The listing builds one solid part. Answer for the finished solid, in the listing's coordinates (mm). Face numbers are marked on the shaded views. A direction names the side the tool comes from. Give positions to 0.01 mm unless a question says otherwise; leave off trailing zeros. Write each loop counter-clockwise with the first axis right and the second up, starting at its lowest first coordinate (ties: lowest second). Pieces come first, ordered by that corner, then holes.
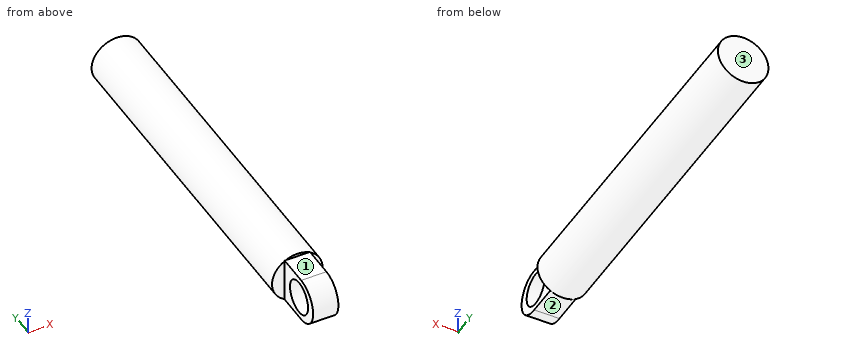
```python
from build123d import *

# Parameters (mm, degrees)
SKETCH5_R           = 14.989713258
BOSS_EXTRUDE3_DEPTH = 200
BOSS_EXTRUDE4_DEPTH = 7.5
SKETCH7_R           = 9.985206203
CUT_EXTRUDE2_DEPTH  = 20


with BuildPart() as part:
    # Sketch5 → Boss-Extrude3 (new body)
    with BuildSketch(Plane(origin=(0, 0, 0), x_dir=(1, 0, 0), z_dir=(0, 1, 0))):
        Circle(SKETCH5_R)
    extrude(amount=BOSS_EXTRUDE3_DEPTH)

    # Sketch6 → Boss-Extrude4 (add, symmetric)
    with BuildSketch(Plane(origin=(0, 0, 0), x_dir=(0, -1, 0), z_dir=(-1, 0, 0))):
        with BuildLine():
            Line((0, 13.292901933), (18.33265387, 13.292901933))
            ThreePointArc((18.33265387, 13.292901933), (31.584492176, -0.298051084), (17.663099627, -13.202315957))
            Line((17.663099627, -13.202315957), (0, -13.202315957))
            Line((0, -13.202315957), (0, 13.292901933))
        make_face()
    extrude(amount=BOSS_EXTRUDE4_DEPTH, both=True)

    # Sketch7 → Cut-Extrude2 (cut, symmetric)
    with BuildSketch(Plane(origin=(7.5, 0, 0), x_dir=(0, 0, -1), z_dir=(1, 0, 0))):
        with Locations((0, -15.988279057)):
            Circle(SKETCH7_R)
    extrude(amount=CUT_EXTRUDE2_DEPTH, both=True, mode=Mode.SUBTRACT)


solid = part.part
```
Item 1: Each of these flat-tipped pins is pushed along its axis until it touches: P1, Ø1, axis at x = -7, z = 8.5, coming from the -Y side; P2, Ø12, axis at y = 37.5, z = 10, coming from the -X side; P3, Ø6, axis at x = -12.5, z = 0.5, coming from the -Y side. Where does it stop, or does it pass through?
Conclusion:
P1: stops at y = -28.93
P2: stops at x = -14.45
P3: stops at y = 0
Item 2: A cutting plane is placed at D-D, the plane x = -11.5. Give the vertices of the cut face in (y, z), plus the area to 3 significant figures.
Conclusion:
outline: (0, -9.61) - (200, -9.61) - (200, 9.61) - (0, 9.61) - close
area: 3,850 mm2
Item 3: Consider probe 1 along Y at (x, z) = (-2.5, 0); probe 2 along Z at (x, y) = (13, 137); probe 3 along Y at (x, z) = (-4, -5). Determine where each line is inside the solid, lowest interval first.
Conclusion:
probe 1: y = -31.59 to -25.97, -6 to 200
probe 2: z = -7.46 to 7.46
probe 3: y = -30.59 to -24.63, -7.35 to 200
Item 4: A cutting plane is placed at A-A, the plane x = 1.75. Give the vertices of the cut face in (y, z).
Conclusion:
outline: (-18.33, 13.29) arc R13.26 ccw (long way) to (-17.66, -13.2) - (0, -13.2) - (0, -14.89) - (200, -14.89) - (200, 14.89) - (0, 14.89) - (0, 13.29) - close; hole circle Ø19.97 at (-15.99, 0)
Item 5: A cutting plane is placed at C-C, the plane y = 106.5. Give the vertices of the cut face in (x, z), plus the area to 3 significant figures.
Conclusion:
outline: circle Ø29.98 at (0, 0)
area: 706 mm2
Item 6: Which of the six approach directions +Z, -Z, +X, -X, +Y, -Y give full straight-line access (tool end or side, diameter ignored) to the marked faces 1, 2 and 3?
Conclusion:
face 1: +Z, +X, -X, -Y
face 2: -Z, +X, -X, -Y
face 3: +Z, -Z, +X, -X, +Y
Item 7: A cutting plane is placed at B-B, the plane z = 0. Give the vertices of the cut face in (x, y).
Conclusion:
outline: (-14.99, 0) - (-7.5, 0) - (-7.5, -6) - (7.5, -6) - (7.5, 0) - (14.99, 0) - (14.99, 200) - (-14.99, 200) - close; (-7.5, -31.59) - (7.5, -31.59) - (7.5, -25.97) - (-7.5, -25.97) - close
